Geometry check sheet. Reference: the model listing, model coordinates, mm. Give positions to 0.01 mm unless a question says otherwise; leave off trailing zeros. Loops run counter-clockwise (first coordinate to the right, second up) from the corner with the lowest first, then second, coordinate; pieces in that order, holes last.
1. Cross-section at C-C, the plane y = 28.5. Record the cut outline in (x, z), plus the area to 3 significant figures.
2. Cross-section at B-B, the plane y = 20. Record the cut outline in (x, z), plus the area to 3 significant figures.
3. Material ranges on L1, parallel to Z at x = 1, y = 29.5; L2, parallel to X at y = 21.5, z = -10; L3, parallel to X at y = 14, z = -18.5, recorded low to high.
4. Cross-section at A-A, the plane x = 0. Record the cut outline in (y, z), plus the area to 3 significant figures.
5. Go/stop test with flat-tipped pins: pin 1 Ø12 at (x, y) = (18.5, 8) entering from -Z; pin 2 Ø8 at (x, z) = (2, 21) entering from +Y (3 decimals); pin 3 Ø16 at (x, y) = (-15, 23.5) entering from -Z. Record where each tip stops, or that it passes through.
6. Cross-section at D-D, the plane y = 3.5. Record the cut outline in (x, z), plus the area to 3 significant figures.
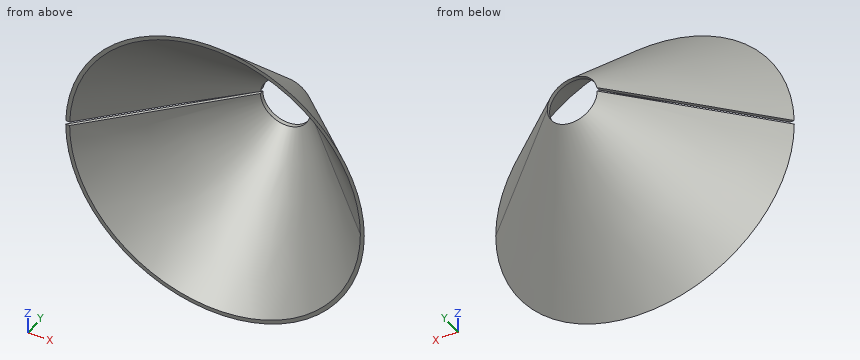
from build123d import *

# Parameters (mm, degrees)
SKETCH3_W          = 6.35
SKETCH3_H          = 17.293961796
CUT_EXTRUDE1_DEPTH = 1


with BuildPart() as part:
    # Sketch1 → Revolve1 (revolve)
    with BuildSketch(Plane.XY):
        Polygon((0, 0), (0, 38), (38, 0), align=None)
    revolve(axis=Axis((0, 0, 0), (0, 1, 0)))

    # Sketch2 → Cut-Revolve1 (revolve, cut)
    with BuildSketch(Plane.XY):
        Polygon((0, 0), (0, 37), (37, 0), align=None)
    revolve(axis=Axis((0, 0, 0), (0, 1, 0)), mode=Mode.SUBTRACT)

    # Sketch3 → Cut-Revolve2 (revolve, cut)
    with BuildSketch(Plane(origin=(0, 0, 0), x_dir=(0, 0, -1), z_dir=(1, 0, 0))):
        with Locations((3.175, 34.250129947)):
            Rectangle(SKETCH3_W, SKETCH3_H)
    revolve(axis=Axis((0, 0, 0), (0, 1, 0)), mode=Mode.SUBTRACT)

    # Sketch15 → Cut-Extrude1 (cut)
    with BuildSketch(Plane.XY):
        Polygon((-39.618894295, 0.734384701), (-37.928802574, -0.95570702), (-4.087663697, 32.885431857), (-5.777755418, 34.575523578), align=None)
    extrude(amount=CUT_EXTRUDE1_DEPTH, mode=Mode.SUBTRACT)


solid = part.part
Result:
1. outline: (-9.5, 0) arc R9.5 ccw (long way) to (-9.45, 1) - (-8.47, 1) - (-8.47, 0.68) arc R8.5 cw (long way) to (-8.5, 0) - close
1. area: 55.6 mm2
2. outline: (-18, 0) arc R18 ccw (long way) to (-17.97, 1) - (-16.97, 1) - (-16.97, 0.96) arc R17 cw (long way) to (-17, 0) - close
2. area: 109 mm2
3. L1: z = -8.44 to -7.43, 7.43 to 8.44
3. L2: x = -13.12 to -11.84, 11.84 to 13.12
3. L3: x = -15.29 to -13.67, 13.67 to 15.29
4. outline: (0, -38) - (31.65, -6.35) - (30.65, -6.35) - (0, -37) - close; (0, 37) - (30.65, 6.35) - (31.65, 6.35) - (0, 38) - close
4. area: 62.3 mm2
5. pin 1: stops at z = -31.64
5. pin 2: stops at y = 20.905
5. pin 3: stops at z = -18.4
6. outline: (-34.5, 0) arc R34.5 ccw (long way) to (-34.49, 1) - (-33.49, 1) arc R33.5 cw (long way) to (-33.5, 0) - close
6. area: 213 mm2
